Part model, mm, in its own coordinate system. A direction names the side the tool comes from. Give positions to 0.01 mm unless a question says otherwise; leave off trailing zeros. Order: outer loops, then holes, each group sorted by start corner. A loop starts at its lowest first (then second) coordinate and runs counter-clockwise, first axis right, second up. Notation, with made-up numbers: M 13,4 L 31,4 A35 ccw 31,42 Z; hole C 20,-3 d1. An arc over 180 degrees is marked long. Answer as a JSON object with one key per item and string values.
Autodesk Fusion 360 part; units mm, degrees
sketch "Sketch1" plane through (0, 0, 0) normal (0, 0, 1) x (1, 0, 0)
  line L0 (0, 0) -> (60, 0)
  line L1 (60, 0) -> (60, -60)
  line L2 (60, -60) -> (0, -60)
  line L3 (0, -60) -> (0, 0)
  dimension "d1" = 60
  dimension "d2" = 60
extrude "Extrude1" add sketch "Sketch1" along normal blind 155
sketch "Sketch2" plane through (0, 0, 0) normal (0, 0, 1) x (1, 0, 0)
  line L0 (0, 0) -> (30, 0)
  line L1 (30, 0) -> (30, -30)
  circle A0 centre (30, -30) radius 27.5
  dimension "d5" = 30
  dimension "d6" = 30
  dimension "d7" = 55
extrude "Extrude2" cut sketch "Sketch2" along normal through all
sketch "Sketch3" plane through (0, 0, 0) normal (1, 0, 0) x (0, 1, 0)
  line L0 (0, 0) -> (0, 5)
  line L1 (0, 5) -> (-10, 5)
  line L2 (-10, 5) -> (-50, 5)
  line L3 (-50, 5) -> (-50, 10)
  line L4 (-50, 10) -> (-10, 10)
  line L5 (-10, 10) -> (-10, 5)
  dimension "d9" = 10
  dimension "d10" = 5
  dimension "d11" = 40
  dimension "d12" = 5
extrude "Extrude3" cut sketch "Sketch3" along normal through all
sketch "Sketch4" plane through (0, 0, 0) normal (-1, 0, 0) x (0, -1, 0)
  line L0 (50, 10) -> (50, 5)
  line L1 (50, 5) -> (10, 5)
  line L2 (10, 5) -> (10, 10)
  line L3 (10, 10) -> (50, 10)
  line L4 (0, 0) -> (60, 0)
  line L5 (60, 0) -> (60, 155)
  line L6 (60, 155) -> (0, 155)
  line L7 (0, 155) -> (0, 0)
  line L8 (0, 155) -> (0.01, 155)
  line L9 (0.01, 155) -> (59.91, 155)
  line L10 (59.91, 155) -> (59.91, 85)
  line L11 (59.91, 85) -> (0.01, 85)
  line L12 (0.01, 85) -> (0.01, 155)
  dimension "d14" = 0.01
  dimension "d15" = 59.9
  dimension "d16" = 70
extrude "Extrude4" add sketch "Sketch4" along normal blind 27 contours L6 L9 L10 L11 L12
sketch "Sketch5" plane through (0, 0, 155) normal (0, 0, 1) x (-1, 0, 0)
  circle A0 centre (-30, 30) radius 27.5
  line L0 (0, 60) -> (-60, 60)
  line L1 (-60, 60) -> (-60, 0)
  line L2 (-60, 0) -> (0, 0)
  line L3 (0, 0) -> (0, 0.01)
  line L4 (0, 0.01) -> (27, 0.01)
  line L5 (27, 0.01) -> (27, 59.91)
  line L6 (27, 59.91) -> (0, 59.91)
  line L7 (0, 59.91) -> (0, 60)
  line L8 (27, 0.01) -> (25, 0.01)
  line L9 (25, 0.01) -> (25, 2.01)
  line L10 (25, 2.01) -> (2, 2.01)
  line L11 (2, 2.01) -> (2, 58.01)
  line L12 (2, 58.01) -> (25, 58.01)
  line L13 (25, 58.01) -> (25, 2.01)
  dimension "d19" = 2
  dimension "d20" = 2
  dimension "d21" = 23
  dimension "d22" = 56
extrude "Extrude5" cut sketch "Sketch5" against normal blind 65 contours L10 L11 L12 L13
sketch "Sketch6" plane through (0, -60, 0) normal (0, -1, 0) x (1, 0, 0)
  line L0 (0, 0) -> (60, 0)
  line L1 (60, 0) -> (60, 155)
  line L2 (60, 155) -> (0, 155)
  line L3 (0, 155) -> (0, 0)
sketch "Sketch7" plane through (60, 0, 0) normal (1, 0, 0) x (0, 1, 0)
  line L0 (-50, 5) -> (-50, 10)
  line L1 (-50, 10) -> (-10, 10)
  line L2 (-10, 10) -> (-10, 5)
  line L3 (-10, 5) -> (-50, 5)
  line L4 (-60, 0) -> (0, 0)
  line L5 (0, 0) -> (0, 155)
  line L6 (0, 155) -> (-60, 155)
  line L7 (-60, 155) -> (-60, 0)
sketch "Sketch8" plane through (0, -60, 0) normal (0, -1, 0) x (1, 0, 0)
sketch "Sketch9" plane through (0, -60, 0) normal (0, -1, 0) x (1, 0, 0)
sketch "Sketch10" plane through (0, 0, 0) normal (0, 1, 0) x (-1, 0, 0)
  line L0 (-60, 0) -> (0, 0)
  line L1 (0, 0) -> (0, 155)
  line L2 (0, 155) -> (-60, 155)
  line L3 (-60, 155) -> (-60, 0)
  line L4 (0, 155) -> (-10.5, 155)
  line L5 (-10.5, 155) -> (-49.5, 155)
  line L6 (-49.5, 155) -> (-49.5, 123)
  line L7 (-49.5, 123) -> (-10.5, 123)
  line L8 (-10.5, 123) -> (-10.5, 155)
  dimension "d25" = 10.5
  dimension "d26" = 39
  dimension "d27" = 32
extrude "Extrude6" add sketch "Sketch10" along normal blind 40 contours L2 L5 L6 L7 L8
sketch "Sketch11" plane through (0, 0, 155) normal (0, 0, 1) x (-1, 0, 0)
  line L0 (2, 2.01) -> (2, 58.01)
  line L1 (2, 58.01) -> (25, 58.01)
  line L2 (25, 58.01) -> (25, 2.01)
  line L3 (25, 2.01) -> (2, 2.01)
  circle A0 centre (-30, 30) radius 27.5
  line L4 (0, 60) -> (-60, 60)
  line L5 (-60, 60) -> (-60, 0)
  line L6 (-60, 0) -> (-49.5, 0)
  line L7 (-49.5, 0) -> (-49.5, -40)
  line L8 (-49.5, -40) -> (-10.5, -40)
  line L9 (-10.5, -40) -> (-10.5, 0)
  line L10 (-10.5, 0) -> (0, 0)
  line L11 (0, 0) -> (0, 0.01)
  line L12 (0, 0.01) -> (27, 0.01)
  line L13 (27, 0.01) -> (27, 59.91)
  line L14 (27, 59.91) -> (0, 59.91)
  line L15 (0, 59.91) -> (0, 60)
sketch "Sketch12" plane through (0, 0, 155) normal (0, 0, 1) x (-1, 0, 0)
sketch "Sketch13" plane through (0, 0, 155) normal (0, 0, 1) x (-1, 0, 0)
sketch "Sketch15" plane through (0, 0, 155) normal (0, 0, 1) x (-1, 0, 0)
  line L0 (-49.5, 0) -> (-47.5, 0)
  line L1 (-47.5, 0) -> (-47.5, -2)
  line L2 (-60, 0) -> (-49.5, 0)
  line L3 (-49.5, 0) -> (-49.5, -40)
  line L4 (-47.5, -2) -> (-12.5, -2)
  line L5 (-12.5, -2) -> (-12.5, -38)
  line L6 (-12.5, -38) -> (-47.5, -38)
  line L7 (-47.5, -38) -> (-47.5, -2)
  dimension "d34" = 2
  dimension "d35" = 2
  dimension "d36" = 35
  dimension "d37" = 36
extrude "Extrude7" cut sketch "Sketch15" against normal blind 30
sketch "Sketch16" plane through (0, 40, 0) normal (0, 1, 0) x (-1, 0, 0)
  line L0 (-10.5, 123) -> (-10.5, 155)
  line L1 (-10.5, 155) -> (-49.5, 155)
  line L2 (-49.5, 155) -> (-49.5, 123)
  line L3 (-49.5, 123) -> (-10.5, 123)
  line L4 (-49.5, 155) -> (-42, 155)
  line L5 (-42, 155) -> (-42, 151)
  line L6 (-42, 151) -> (-18, 151)
  line L7 (-18, 151) -> (-18, 127)
  line L8 (-18, 127) -> (-42, 127)
  line L9 (-42, 127) -> (-42, 151)
  dimension "d40" = 7.5
  dimension "d41" = 4
  dimension "d42" = 24
  dimension "d43" = 24
extrude "Extrude8" cut sketch "Sketch16" against normal blind 15 contours L6 L7 L8 L9
sketch "Sketch17" plane through (0, 2, 0) normal (0, 1, 0) x (-1, 0, 0)
  line L0 (-12.5, 155) -> (-47.5, 155)
  line L1 (-47.5, 155) -> (-47.5, 125)
  line L2 (-47.5, 125) -> (-12.5, 125)
  line L3 (-12.5, 125) -> (-12.5, 155)
  line L4 (-47.5, 155) -> (-28, 155)
  line L5 (-28, 155) -> (-28, 139)
  circle A0 centre (-28, 139) radius 5
  dimension "d46" = 19.5
  dimension "d47" = 16
  dimension "d48" = 10
extrude "Extrude9" cut sketch "Sketch17" against normal blind 12 contours A0
sketch "Sketch18" plane through (0, -60, 0) normal (0, -1, 0) x (1, 0, 0)
sketch "Sketch19" plane through (0, -60, 0) normal (0, -1, 0) x (1, 0, 0)
sketch "Sketch20" plane through (0, -60, 0) normal (0, -1, 0) x (1, 0, 0)
  line L0 (45.5, 105) -> (14.5, 105)
  line L1 (14.5, 105) -> (14.5, 54)
  line L2 (14.5, 54) -> (45.5, 54)
  line L3 (45.5, 54) -> (45.5, 105)
  line L4 (60, 0) -> (60, 155)
  line L5 (45.5, 105) -> (60, 105)
  line L6 (60, 105) -> (60, 155)
  dimension "d52" = 31
  dimension "d53" = 51
  dimension "d96" = 50
  dimension "d97" = 14.5
extrude "Extrude10" add sketch "Sketch20" along normal blind 22
sketch "Sketch21" plane through (0, 0, 155) normal (0, 0, 1) x (-1, 0, 0)
  line L0 (-12.5, -2) -> (-12.5, -38)
  line L1 (-12.5, -38) -> (-47.5, -38)
  line L2 (-47.5, -38) -> (-47.5, -2)
  line L3 (-47.5, -2) -> (-12.5, -2)
  line L4 (2, 2.01) -> (2, 58.01)
  line L5 (2, 58.01) -> (25, 58.01)
  line L6 (25, 58.01) -> (25, 2.01)
  line L7 (25, 2.01) -> (2, 2.01)
  circle A0 centre (-30, 30) radius 27.5
  line L8 (0, 60) -> (-60, 60)
  line L9 (-60, 60) -> (-60, 0)
  line L10 (-60, 0) -> (-49.5, 0)
  line L11 (-49.5, 0) -> (-49.5, -40)
  line L12 (-49.5, -40) -> (-10.5, -40)
  line L13 (-10.5, -40) -> (-10.5, 0)
  line L14 (-10.5, 0) -> (0, 0)
  line L15 (0, 0) -> (0, 0.01)
  line L16 (0, 0.01) -> (27, 0.01)
  line L17 (27, 0.01) -> (27, 59.91)
  line L18 (27, 59.91) -> (0, 59.91)
  line L19 (0, 59.91) -> (0, 60)
  line L20 (-14.5, 82) -> (-14.5, 80)
  line L21 (-14.5, 80) -> (-16.5, 80)
  dimension "d56" = 2
  dimension "d57" = 2
sketch "Sketch22" plane through (0, 0, 155) normal (0, 0, 1) x (-1, 0, 0)
  line L0 (-16.5, 80) -> (-43.5, 80)
  line L1 (-43.5, 80) -> (-43.5, 62)
  line L2 (-43.5, 62) -> (-16.5, 62)
  line L3 (-16.5, 62) -> (-16.5, 80)
  dimension "d58" = 27
  dimension "d59" = 18
extrude "Extrude11" cut sketch "Sketch22" against normal blind 99
sketch "Sketch23" plane through (0, 0, 155) normal (0, 0, 1) x (-1, 0, 0)
sketch "Sketch24" plane through (0, 0, 155) normal (0, 0, 1) x (1, 0, 0)
sketch "Sketch26" plane through (-2, 0, 0) normal (-1, 0, 0) x (0, -1, 0)
  line L0 (58.01, 155) -> (2.01, 155)
  line L1 (2.01, 155) -> (2.01, 90)
  line L2 (2.01, 90) -> (58.01, 90)
  line L3 (58.01, 90) -> (58.01, 155)
  line L4 (2.01, 155) -> (2.01, 153)
  line L5 (2.01, 153) -> (7.01, 153)
  line L6 (7.01, 153) -> (17.01, 153)
  line L7 (17.01, 153) -> (17.01, 93)
  line L8 (17.01, 93) -> (7.01, 93)
  line L9 (7.01, 93) -> (7.01, 153)
  line L10 (30.01, 155) -> (30.01, 90)
  line L11 (2.01, 155) -> (58.01, 155)
  line L12 (43.01, 153) -> (43.01, 93)
  line L13 (53.01, 153) -> (43.01, 153)
  line L14 (53.01, 93) -> (53.01, 153)
  line L15 (43.01, 93) -> (53.01, 93)
  dimension "d66" = 2
  dimension "d67" = 5
  dimension "d68" = 10
  dimension "d69" = 60
extrude "Extrude14" cut sketch "Sketch26" against normal blind 25 contours L12 L13 L14 L15
extrude "Extrude13" cut sketch "Sketch26" against normal blind 25 contours L6 L7 L8 L9
sketch "Sketch27" plane through (60, 0, 0) normal (1, 0, 0) x (0, 1, 0)
  line L0 (-60, 155) -> (-50, 155)
  line L1 (-50, 155) -> (-10, 155)
  line L2 (-10, 155) -> (-10, 110)
  line L3 (-10, 110) -> (-50, 110)
  line L4 (-50, 110) -> (-50, 155)
  dimension "d74" = 10
  dimension "d75" = 40
  dimension "d76" = 45
extrude "Extrude15" cut sketch "Sketch27" against normal blind 20
sketch "Sketch28" plane through (0, 0, 155) normal (0, 0, 1) x (-1, 0, 0)
  line L0 (-60, 30) -> (0, 30) construction
  line L1 (-60, 60) -> (-60, 0)
  line L2 (0, 30) -> (0, 25)
  line L3 (0, 25) -> (-60, 25)
  line L4 (-60, 25) -> (-60, 81)
  line L5 (-60, 81) -> (0, 81)
  line L6 (0, 81) -> (0, 25)
  dimension "d79" = 5
  dimension "d80" = 60
  dimension "d81" = 56
extrude "Extrude16" add sketch "Sketch28" along normal blind 30
sketch "Sketch29" plane through (0, 0, 155) normal (0, 0, 1) x (-1, 0, 0)
sketch "Sketch30" plane through (0, 0, 0) normal (-1, 0, 0) x (0, -1, 0)
  line L0 (59.91, 155) -> (59.91, 85)
  line L1 (59.91, 85) -> (0.01, 85)
  line L2 (0.01, 85) -> (0.01, 155)
  line L3 (0.01, 155) -> (0, 155)
  line L4 (0, 155) -> (0, 0)
  line L5 (0, 0) -> (60, 0)
  line L6 (60, 0) -> (60, 155)
  line L7 (60, 155) -> (81, 155)
  line L8 (81, 155) -> (81, 185)
  line L9 (81, 185) -> (25, 185)
  line L10 (25, 185) -> (25, 155)
  line L11 (25, 155) -> (59.91, 155)
  line L12 (50, 10) -> (50, 5)
  line L13 (50, 5) -> (10, 5)
  line L14 (10, 5) -> (10, 10)
  line L15 (10, 10) -> (50, 10)
  line L16 (25, 185) -> (28, 185)
  line L17 (28, 185) -> (28, 182)
  line L18 (28, 182) -> (78, 182)
  line L19 (78, 182) -> (78, 158)
  line L20 (78, 158) -> (28, 158)
  line L21 (28, 158) -> (28, 182)
  dimension "d84" = 3
  dimension "d85" = 3
  dimension "d86" = 50
  dimension "d87" = 24
extrude "Extrude17" cut sketch "Sketch30" against normal through all contours L18 L19 L20 L21
sketch "Sketch31" plane through (60, 0, 0) normal (1, 0, 0) x (0, 1, 0)
sketch "Sketch32" plane through (0, 0, 185) normal (0, 0, 1) x (-1, 0, 0)
  line L0 (0, 81) -> (-60, 81)
  line L1 (-60, 81) -> (-60, 25)
  line L2 (-60, 25) -> (0, 25)
  line L3 (0, 25) -> (0, 81)
  line L4 (0, 25) -> (-60, 25)
  line L5 (-60, 25) -> (-60, 48)
  line L6 (-60, 48) -> (0, 48)
  line L7 (0, 48) -> (0, 25)
  dimension "d89" = 60
  dimension "d90" = 23
sketch "Sketch33" plane through (0, 0, 158) normal (0, 0, 1) x (-1, 0, 0)
  line L0 (-60, 78) -> (-60, 28)
  line L1 (-60, 28) -> (0, 28)
  line L2 (0, 28) -> (0, 78)
  line L3 (0, 78) -> (-60, 78)
  line L4 (0, 28) -> (-5, 28)
  line L5 (-5, 28) -> (-53, 28)
  line L6 (-53, 28) -> (-53, 40)
  line L7 (-53, 40) -> (-5, 40)
  line L8 (-5, 40) -> (-5, 28)
  dimension "d93" = 48
  dimension "d94" = 12
extrude "Extrude19" cut sketch "Sketch33" against normal through all contours L1 L5 L6 L7 L8
equation "d60 = -49.00 mm - 50 mm"
1. Cut at B-B on z = 162.5. Give the cut face in (x, y).
Worked answers:
{"outline": "M 0,-81 L 60,-81 L 60,-78 L 0,-78 Z; M 0,-28 L 60,-28 L 60,-25 L 0,-25 Z"}
2. Pin check, flat tips, straight feed: P1, Ø8, axis at x = 31.5, z = 100, coming from the +Y side; P2, Ø0.6, axis at x = 34, y = 39, coming from the +Z side; P3, Ø6, axis at x = 4.5, z = 145.5, coming from the -Y side. Stop position of each tip, or through.
Worked answers:
{"P1": "stops at y = 0", "P2": "stops at z = 155", "P3": "stops at y = -60"}
3. Cut at A-A on y = -30. State how many separate pieces and enclosed holes the cut face has, plus the area to 3 significant figures.
Worked answers:
{"separate pieces": "6", "enclosed holes": "0", "area": "1,250 mm^2"}
4. Two-plate mould, pull along X, no slides. Class faces 1 (the flat face through (-13, -0.01, 120)), 2 (the flat face through (2, -43.01, 123)), 3 (the flat face through (45.5, -71, 79)): +X half, -X half, draft (parallel to the pull), parting line (faces both ways), or undercut.
Worked answers:
{"face 1": "draft", "face 2": "undercut", "face 3": "+X half"}
5. Cut at C-C on y = -66.5. Give the cut face in (x, z).
Worked answers:
{"outline": "M 0,155 L 60,155 L 60,158 L 0,158 Z; M 0,182 L 60,182 L 60,185 L 0,185 Z; M 14.5,54 L 45.5,54 L 45.5,105 L 43.5,105 L 43.5,56 L 16.5,56 L 16.5,105 L 14.5,105 Z"}
6. Which spindle directions (+Z, -Z, +X, -X, +Y, -Y) get a long thin tool onto all of the face, cutting with end or side? Do faces 4 (the flat face through (2, -30, 5)), 5 (the flat face through (-14, -2.01, 123)), 6 (the cylindrical face through (56.23, -38.26, 76.41)), 7 (the cylindrical face through (23.381, -0.665, 137.085)), 8 (the flat face through (4, -11, 153)). Say none if no direction does.
Worked answers:
{"face 4": "+X, -X", "face 5": "+Z", "face 6": "-Z", "face 7": "+Y", "face 8": "none"}
7. Cut at D-D on x = -18. Give the cut face in (y, z), plus the area to 3 significant figures.
Worked answers:
{"outline": "M -59.91,85 L -0.01,85 L -0.01,155 L -2.01,155 L -2.01,90 L -58.01,90 L -58.01,155 L -59.91,155 Z", "area": "553 mm^2"}
8. Probe line 1 along Y through (x, z) = (29, 80); line 2 along X through (y, z) = (-2.2, 139); line 3 along Z through (x, y) = (28, 0.75). List the from-to ranges inside material, lowest first.
Worked answers:
{"line 1": "y = -82 to -80, -62 to -57.48, -2.52 to 0", "line 2": "x = -27 to -25, -2 to 23, 33 to 60", "line 3": "z = 123 to 134, 144 to 155"}
